Source: CAD feature listing. Evaluate the final solid. Frame: model axes, mm. A direction names the side the tool comes from. Round coordinates to 2 decimals unless told otherwise and drop trailing zeros. Order: outer loops, then holes, each group sorted by start corner. A loop starts at its lowest first (then second) coordinate and runs counter-clockwise, first axis right, second up. Notation, with made-up numbers: (-37, -3) -> (21, -3) arc R7 cw to (21, 5) -> close; hole circle Ø4 at (50, -34.75). An arc over 180 degrees is marked (long way). One line per item, written item: value. Start each with the question number.
1) Pin query (flat end, axial travel): P1, Ø6, axis at x = 4, y = -60, coming from the -Z side; P2, Ø8, axis at x = 5, y = -65, coming from the +Z side; P3, Ø1.2, axis at x = -5, y = -77, coming from the -Z side. Return the tip coordinate at first contact, or that it passes through.
2) Section D-D (z = -3). Return the cut outline in (x, y).
3) Mould query, pull axis Y, two halves, no side actions, for faces 5 (the face through (-3, -78, -2)), 6 (the face through (-2.529, -64.99, -3.488)), 7 (the face through (-12.669, -69, -1)), 8 (the face through (-2.53, -66.64, -1.29)). Classes: pulls with the +Y half, pulls with the -Y half, needs draft (parallel to the pull), parting line crosses it, or undercut.
4) Section B-B (x = -5.25). Return the cut outline in (y, z).
5) Section A-A (z = -1.5). Return the cut outline in (x, y).
6) Reachability of faces 1 (the face through (-2.8, -77.4, -4)), 2 (the face through (-2.53, -53.15, -6.99)), 3 (the face through (-2.5, -78.4, 0)), 4 (the face through (-7.6, -79.5, -2.4)) from +Z, -Z, +X, -X, +Y, -Y: full face, straight path, thin tool, end or side. Return the list, or none.
7) Ray query, L1, parallel to Z at x = 3.5, y = -64.75; L2, parallel to Z at x = 3.75, y = -61.5. Return the intervals inside material, ascending.
8) Section C-C (y = -74.5). Return the cut outline in (x, z), and give its area (3 significant figures).
```python
from build123d import *

# Parameters (mm, degrees)
CROQUIS1_W                = 20
CROQUIS1_H                = 1.1
SALIENTE_EXTRUIR1_DEPTH   = 4
SALIENTE_EXTRUIR1_2_DEPTH = 4
CORTAR_EXTRUIR1_DEPTH     = 1.1
SALIENTE_EXTRUIR2_DEPTH   = 20


with BuildPart() as part:
    # Croquis1 → Saliente-Extruir1 (new body)
    with BuildSketch(Plane.XY):
        with Locations((-2.668808514, -79.450421588)):
            Rectangle(CROQUIS1_W, CROQUIS1_H)
    extrude(amount=-SALIENTE_EXTRUIR1_DEPTH)

    # Croquis2 → Cortar-Extruir1 (cut)
    with BuildSketch(Plane.XZ.offset(80.000421588)):
        Polygon((8.185712697, -4), (-2.668808514, -1.066345619), (-13.523329725, -4), align=None)
    extrude(amount=-CORTAR_EXTRUIR1_DEPTH, mode=Mode.SUBTRACT)



with BuildPart() as body_2:
    # Croquis1 → Saliente-Extruir1 2 (new body)
    with BuildSketch(Plane.XY):
        with Locations((-2.668808514, -77.450421588)):
            Rectangle(CROQUIS1_W, CROQUIS1_H)
    extrude(amount=-SALIENTE_EXTRUIR1_2_DEPTH)


with BuildPart() as part_1:
    add(part.part)

    add(body_2.part)  # Saliente-Extruir2 merges body 2
    # Croquis3 → Saliente-Extruir2 (add, through all)
    with BuildSketch(Plane(origin=(7.331191486, 0, 0), x_dir=(0, 0, -1), z_dir=(1, 0, 0))):
        Polygon((0, -76.900421588), (0, -80.000421588), (-3.57176217, -80.000421588), (6.293776867, -52.895075854), (7.703315798, -53.408106069), (-0.847187785, -76.900421588), align=None)
    extrude(amount=-SALIENTE_EXTRUIR2_DEPTH)


solid = part_1.part
```
Findings:
1. P1: z = -6.4
1. P2: z = -0.43
1. P3: z = -4
2. outline: (-12.67, -80) -> (-9.82, -80) -> (-9.82, -78.9) -> (-12.67, -78.9) -> close; (-12.67, -78) -> (7.33, -78) -> (7.33, -76.9) -> (-12.67, -76.9) -> close; (-12.67, -66.33) -> (7.33, -66.33) -> (7.33, -61.94) -> (-12.67, -61.94) -> close; (4.49, -80) -> (7.33, -80) -> (7.33, -78.9) -> (4.49, -78.9) -> close
3. face 5: undercut
3. face 6: undercut
3. face 7: needs draft
3. face 8: pulls with the +Y half
4. outline: (-80, -1.76) -> (-78.9, -1.76) -> (-78.9, 0) -> (-78, 0) -> (-78, -4) -> (-76.9, -4) -> (-76.9, 0.85) -> (-53.41, -7.7) -> (-52.9, -6.29) -> (-80, 3.57) -> close
5. outline: (-12.67, -80) -> (-4.27, -80) -> (-4.27, -78.9) -> (-12.67, -78.9) -> close; (-12.67, -78) -> (7.33, -78) -> (7.33, -76.9) -> (-12.67, -76.9) -> close; (-12.67, -70.45) -> (7.33, -70.45) -> (7.33, -66.07) -> (-12.67, -66.07) -> close; (-1.06, -80) -> (7.33, -80) -> (7.33, -78.9) -> (-1.06, -78.9) -> close
6. face 1: -Z, +X, -X, -Y
6. face 2: -Z, +X, -X, +Y
6. face 3: -Z, +X, -X
6. face 4: -Z, -Y
7. L1: -3.58 to -1.98
7. L2: -4.76 to -3.16
8. outline: (-12.67, -0.03) -> (7.33, -0.03) -> (7.33, 1.57) -> (-12.67, 1.57) -> close
8. area: 31.9 mm2
